Can you work these out from the drawing? Everything is in mm from the part's minimum corner. Coordinates: 2 decimals unless noted, no trailing zeros. Write each loop counter-clockwise with the first axis right and the second up, starting at its lowest first coordinate (ties: lowest second). Pieces come first, ordered by that corner, then holes. Notation, with made-up numbers: (79, -37) -> (126, -37) arc R11 cw to (126, -22) -> close; hole circle Ø11 at (-39, 59). An arc over 180 degrees is marked (long way). Answer as CSV lines item,"result". Start each with the question number.
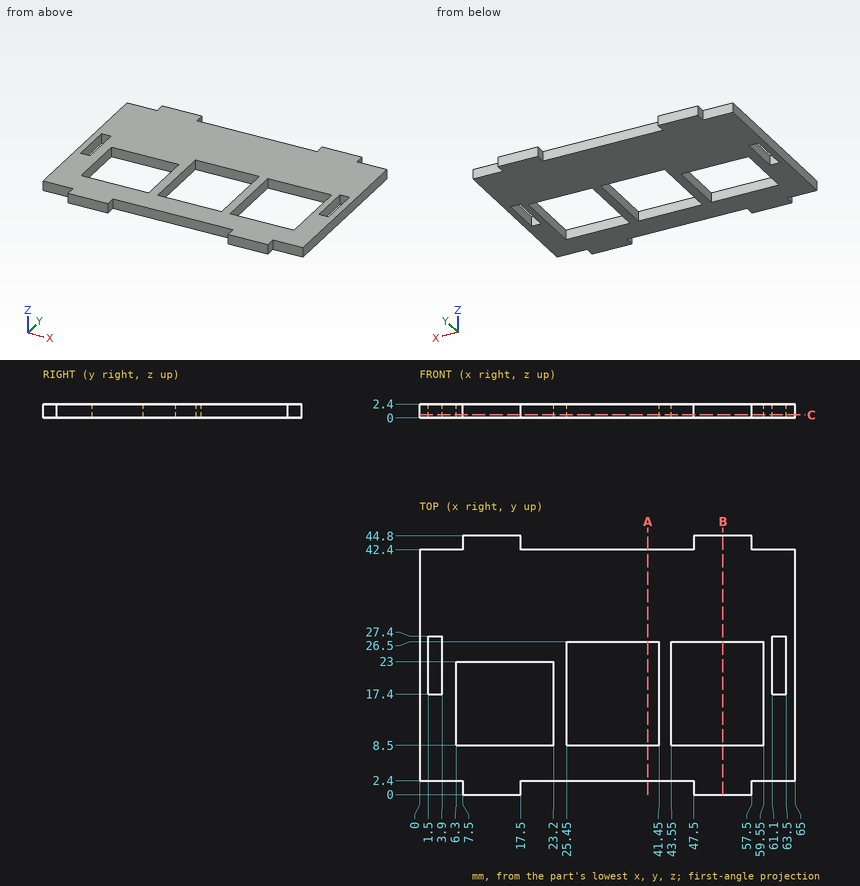
Q1. Imagine slicing it at A-A (x = 39.5). Write out the boundary of the cut face in (y, z).
Q2. Imagine slicing it at C-C (z = 0.5). State how many separate pieces and enclosed holes the cut face has, then the cut area to 3 significant figures.
Q3. I need wall thicknesses on L1, parallel to X at y = 26, z = 1.65; L2, parallel to Y at x = 21.5, z = 0.35; L3, parallel to Y at x = 28, z = 1.55. Which ranges of each line are inside material? Lowest first, please.
Q4. For pin 1 (0.7 mm diameter, centred on x = 3, z = 1.5, fed in from +Y); pin 2 (4 mm diameter, centred on x = 33, y = 38, fed in from -Z); pin 3 (0.7 mm diameter, centred on y = 43.5, z = 1.5, fed in from -X); pin 4 (0.7 mm diameter, centred on x = 5.5, z = 1.5, fed in from -Y), each with a flat end and sliding along its axis, tell me the tip position at first contact or that it passes through.
Q5. Imagine slicing it at B-B (x = 52.5). Write out the boundary of the cut face in (y, z).
Entries:
1,outline,"(2.4, 0) -> (8.5, 0) -> (8.5, 2.4) -> (2.4, 2.4) -> close; (26.5, 0) -> (42.4, 0) -> (42.4, 2.4) -> (26.5, 2.4) -> close"
2,separate pieces,"1"
2,enclosed holes,"5"
2,area,"1,830 mm2"
3,L1,"0 to 1.5, 3.9 to 25.45, 41.45 to 43.55, 59.55 to 61.1, 63.5 to 65"
3,L2,"2.4 to 8.5, 23 to 42.4"
3,L3,"2.4 to 8.5, 26.5 to 42.4"
4,pin 1,"y = 42.4"
4,pin 2,"z = 0"
4,pin 3,"x = 7.5"
4,pin 4,"y = 2.4"
5,outline,"(0, 0) -> (8.5, 0) -> (8.5, 2.4) -> (0, 2.4) -> close; (26.5, 0) -> (44.8, 0) -> (44.8, 2.4) -> (26.5, 2.4) -> close"
